from build123d import *

# Parameters (mm, degrees)
F0_R      = 5
F0_R_2    = 10
F1_DEPTH  = 11
F2_R      = 14
F2_R_2    = 10
F3_DEPTH  = 22.3
F4_R      = 30
F4_R_2    = 25
F5_DEPTH  = 14.5
F6_R      = 5
F7_DEPTH  = 8
F8_R      = 25
F8_R_2    = 10
F9_DEPTH  = 2.3
F10_R     = 24.5
F10_R_2   = 14.5
F11_DEPTH = 14
F12_R     = 1.5


with BuildPart() as f1:
    # F0 (on Front) → F1 (new body)
    with BuildSketch(Plane.XZ):
        with BuildLine():
            ThreePointArc((-10.48323, 49.727778), (-2.417938, 33.757066), (11.5, 45))
            ThreePointArc((11.5, 45), (11.242934, 47.417938), (10.48323, 49.727778))
            ThreePointArc((10.48323, 49.727778), (0, 56.5), (-10.48323, 49.727778))
        make_face()
        with Locations((0, 45)):
            Circle(F0_R, mode=Mode.SUBTRACT)
        with BuildLine():
            ThreePointArc((10.48323, 49.727778), (11.242934, 47.417938), (11.5, 45))
            ThreePointArc((11.5, 45), (-2.417938, 33.757066), (-10.48323, 49.727778))
            Line((-10.48323, 49.727778), (-27.347557, 12.333333))
            ThreePointArc((-27.347557, 12.333333), (0, 30), (27.347557, 12.333333))
            Line((27.347557, 12.333333), (10.48323, 49.727778))
        make_face()
        with BuildLine():
            ThreePointArc((30, 0), (29.329394, 6.307665), (27.347557, 12.333333))
            ThreePointArc((27.347557, 12.333333), (0, 30), (-27.347557, 12.333333))
            ThreePointArc((-27.347557, 12.333333), (-30, 0), (-27.347557, -12.333333))
            ThreePointArc((-27.347557, -12.333333), (0, -30), (27.347557, -12.333333))
            ThreePointArc((27.347557, -12.333333), (29.329394, -6.307665), (30, 0))
        make_face()
        Circle(F0_R_2, mode=Mode.SUBTRACT)
        with BuildLine():
            ThreePointArc((27.347557, -12.333333), (0, -30), (-27.347557, -12.333333))
            Line((-27.347557, -12.333333), (-10.48323, -49.727778))
            ThreePointArc((-10.48323, -49.727778), (-2.417938, -33.757066), (11.5, -45))
            ThreePointArc((11.5, -45), (11.242934, -47.417938), (10.48323, -49.727778))
            Line((10.48323, -49.727778), (27.347557, -12.333333))
        make_face()
        with BuildLine():
            ThreePointArc((11.5, -45), (-2.417938, -33.757066), (-10.48323, -49.727778))
            ThreePointArc((-10.48323, -49.727778), (0, -56.5), (10.48323, -49.727778))
            ThreePointArc((10.48323, -49.727778), (11.242934, -47.417938), (11.5, -45))
        make_face()
        with Locations((0, -45)):
            Circle(F0_R, mode=Mode.SUBTRACT)
    extrude(amount=F1_DEPTH)

    # F2 (on face) → F3 (join)
    with BuildSketch(Plane.XZ.offset(11)):
        Circle(F2_R)
        Circle(F2_R_2, mode=Mode.SUBTRACT)
    extrude(amount=F3_DEPTH)

    # F4 (on face) → F5 (join)
    with BuildSketch(Plane.XZ.offset(11)):
        Circle(F4_R)
        Circle(F4_R_2, mode=Mode.SUBTRACT)
    extrude(amount=F5_DEPTH)

    # F6 (on face) → F7 (join)
    with BuildSketch(Plane.XZ.offset(11)):
        with BuildLine():
            ThreePointArc((-11.5, 45), (0, 33.5), (11.5, 45))
            ThreePointArc((11.5, 45), (11.242934, 47.417938), (10.48323, 49.727778))
            ThreePointArc((10.48323, 49.727778), (0, 56.5), (-10.48323, 49.727778))
            ThreePointArc((-10.48323, 49.727778), (-11.242934, 47.417938), (-11.5, 45))
        make_face()
        with Locations((0, 45)):
            Circle(F6_R, mode=Mode.SUBTRACT)
        with BuildLine():
            Line((11.5, 27.708302), (11.5, 45))
            ThreePointArc((11.5, 45), (0, 33.5), (-11.5, 45))
            Line((-11.5, 45), (-11.5, 27.708302))
            ThreePointArc((-11.5, 27.708302), (0, 30), (11.5, 27.708302))
        make_face()
        with BuildLine():
            ThreePointArc((11.5, -27.708302), (0, -30), (-11.5, -27.708302))
            Line((-11.5, -27.708302), (-11.5, -45))
            ThreePointArc((-11.5, -45), (0, -33.5), (11.5, -45))
            Line((11.5, -45), (11.5, -27.708302))
        make_face()
        with BuildLine():
            ThreePointArc((11.5, -45), (0, -33.5), (-11.5, -45))
            ThreePointArc((-11.5, -45), (0, -56.5), (11.5, -45))
        make_face()
        with Locations((0, -45)):
            Circle(F6_R, mode=Mode.SUBTRACT)
    extrude(amount=F7_DEPTH)

    # F8 (on face) → F9 (cut)
    with BuildSketch(Plane(origin=(0, 0, 0), x_dir=(-1, 0, 0), z_dir=(0, 1, 0))):
        Circle(F8_R)
        Circle(F8_R_2, mode=Mode.SUBTRACT)
    extrude(amount=-F9_DEPTH, mode=Mode.SUBTRACT)

    # F10 (on face) → F11 (join)
    with BuildSketch(Plane.XZ.offset(11)):
        Circle(F10_R)
        Circle(F10_R_2, mode=Mode.SUBTRACT)
    extrude(amount=F11_DEPTH)

    # F12
    f12_edges = [f1.edges().sort_by_distance(p)[0] for p in [
        (-24.5, -25, 0),
        (-14.5, -25, 0),
    ]]
    fillet(f12_edges, radius=F12_R)


solid = f1.part
Design review of the part built by this model. Coordinates are the model's own, in mm. A direction names the side the tool comes from. Give positions to 0.01 mm unless a question says otherwise; leave off trailing zeros. Order: outer loops, then holes, each group sorted by start corner. A loop starts at its lowest first (then second) coordinate and runs counter-clockwise, first axis right, second up. Notation, with made-up numbers: (19.5, 65.25) - (28.5, 65.25) arc R11 cw to (28.5, 83.25) - close; hole circle Ø5 at (-13, 31.5). An arc over 180 degrees is marked (long way). Use CSV: the item, a comma, the result in double quotes. Start each with the question number.
Q1. Take a section at D-D (y = -6.5). State the section outline as (x, z) points.
Q2. Machinability: for faces 1 (the face through (11.5, -15, -36)), 2 (the face through (-7, -25.5, 25)), 3 (the face through (-16, -11, 31)), 4 (the face through (-16, -11, -31)), which of the approach directions +Z, -Z, +X, -X, +Y, -Y give a long, thin tool a straight path to every point of the face, cutting with its end or side? Answer none if there is none.
Q3. Take a section at B-B (y = -21). State the section outline as (x, z) points, and give its area (3 significant figures).
Q4. Take a section at A-A (y = -12.5). State the section outline as (x, z) points.
Q5. Take a section at C-C (x = 0). Count the separate pieces of the cut face and the enclosed holes in it, and give its area (3 significant figures).
Q6. Draft analysis for pull direction X (two halves, no side actions). For faces 5 (the face through (-23.846, -1.134, 7.509)), 6 (the face through (16, -11, 31)), 7 (the face through (18.8, -5.42, -31.29)), state which applies: pulls with the +X half, pulls with the -X half, needs draft (parallel to the pull), parting line crosses it, or undercut.
Q7. For P1, Ø5, axis at x = -9.5, z = -29.5, coming from the +Y side; P2, Ø5, axis at x = 15, z = -38, coming from the -Y side; P3, Ø2.5, axis at y = -15, z = -35, coming from the -X side; P4, Ø18.5, axis at x = 17, z = 26.5, coming from the -Y side, all flat-tipped, find the tip position at first contact; note any pin that passes through.
Q8. For line 1 (Z direction, x = 0, y = -20); line 2 (Z direction, x = 0, y = -9.5); line 3 (Z direction, x = 4, y = -24), list the stretches that pass through material, from the lowest coordinate up.
Calculated:
1,outline,"(-27.35, -12.33) - (-10.48, -49.73) arc R11.5 ccw to (10.48, -49.73) - (27.35, -12.33) arc R30 ccw to (30, 0) arc R30 ccw to (27.35, 12.33) - (10.48, 49.73) arc R11.5 ccw to (-10.48, 49.73) - (-27.35, 12.33) arc R30 ccw to start; hole circle Ø20 at (0, 0); hole circle Ø10 at (0, -45); hole circle Ø10 at (0, 45)"
2,face 1,"-Z, +X, -Y"
2,face 2,"-Y"
2,face 3,"+Z, -X, -Y"
2,face 4,"-Z, -X, -Y"
3,outline,"circle Ø60 at (0, 0); circle Ø49 at (0, 0); circle Ø28 at (0, 0); hole circle Ø50 at (0, 0); hole circle Ø29 at (0, 0); hole circle Ø20 at (0, 0)"
3,area,"2,390 mm²"
4,outline,"circle Ø49 at (0, 0); circle Ø28 at (0, 0); (-11.5, -45) arc R11.5 ccw to (11.5, -45) - (11.5, -27.71) arc R30 ccw to (11.5, 27.71) - (11.5, 45) arc R11.5 ccw to (10.48, 49.73) arc R11.5 ccw to (-10.48, 49.73) arc R11.5 ccw to (-11.5, 45) - (-11.5, 27.71) arc R30 ccw to (-11.5, -27.71) - close; hole circle Ø50 at (0, 0); hole circle Ø29 at (0, 0); hole circle Ø20 at (0, 0); hole circle Ø10 at (0, -45); hole circle Ø10 at (0, 45)"
5,separate pieces,"4"
5,enclosed holes,"0"
5,area,"1,600 mm²"
6,face 5,"undercut"
6,face 6,"needs draft"
6,face 7,"pulls with the +X half"
7,P1,"stops at y = 0"
7,P2,"stops at y = -11"
7,P3,"stops at x = -11.5"
7,P4,"stops at y = -25.5"
8,line 1,"z = -30 to -25, -24.5 to -14.5, -14 to -10, 10 to 14, 14.5 to 24.5, 25 to 30"
8,line 2,"z = -56.5 to -50, -40 to -10, 10 to 40, 50 to 56.5"
8,line 3,"z = -29.73 to -24.68, -24.08 to -14.03, -13.42 to -9.17, 9.17 to 13.42, 14.03 to 24.08, 24.68 to 29.73"
